Could you check a few things on this model? Use its own coordinates, in mm. Coordinates: 2 decimals unless noted, no trailing zeros. Order: outer loops, then holes, each group sorted by start corner. A loop starts at its lowest first (then second) coordinate and runs counter-clockwise, first axis right, second up. Notation, with made-up numbers: (39, 68) - (83, 68) arc R24 ccw to (83, 88) - close; hole circle Ø4 at (17.5, 39.25). An arc over 180 degrees is marked (long way). One line per item, written item: value. Start each with the question number.
from build123d import *

# Parameters (mm, degrees)
F0_R     = 13.75
F0_R_2   = 11.25
F1_DEPTH = 110
F4_R     = 5
F5_DEPTH = 33.751
F6_DEPTH = 33.751


with BuildPart() as f1:
    # F0 (on Front) → F1 (new body)
    with BuildSketch(Plane.XZ):
        Circle(F0_R)
        Circle(F0_R_2, mode=Mode.SUBTRACT)
    extrude(amount=F1_DEPTH)

    # F4 (on offset) → F5 (cut, through all)
    with BuildSketch(Plane.XY.offset(-20)):
        with Locations((0, -30)):
            Circle(F4_R)
    extrude(amount=F5_DEPTH, mode=Mode.SUBTRACT)

    # F4 (on offset) → F6 (cut, through all)
    with BuildSketch(Plane.XY.offset(-20)):
        with BuildLine():
            Line((-21.2415, 7.674746), (-21.2415, -2.517288))
            Line((-21.2415, -2.517288), (-21.2415, -5.328869))
            ThreePointArc((-21.2415, -5.328869), (0.089579, -8.9e-05), (21.399274, -5.413752))
            Line((21.399274, -5.413752), (21.399274, -2.555365))
            Line((21.399274, -2.555365), (21.399274, 6.795851))
            Line((21.399274, 6.795851), (-21.2415, 7.674746))
        make_face()
    extrude(amount=F6_DEPTH, mode=Mode.SUBTRACT)


solid = f1.part
Q1. I'm going to push flat-ended pins straight in: pin 1 (2 mm diameter, centred on x = -9, y = -68.5, fed in from +Z); pin 2 (12 mm diameter, centred on x = 9.5, y = -94, fed in from +Z); pin 3 (8 mm diameter, centred on x = 7.5, z = -5.5, fed in from +Y); pin 4 (8 mm diameter, centred on x = 0, y = -30, fed in from +Z). Where does each tip first touch, or does it pass through?
Q2. I want a section at D-D on y = -10. Please give me the cut outline in (x, z).
Q3. We'd pull the mould along Y, two halves only. Please class faces 1 (the cylindrical face through (5.1, -0.29, -10.25)), 2 (the cylindrical face through (3, -26, -12)), 3 (the cylindrical face through (10.39, -54.23, -4.31)): +Y half, -Y half, draft (parallel to the pull), parting line (faces both ways), or undercut.
Q4. If I drill on L1, parallel to Y at x = 0, z = -12.4; L2, parallel to Z at x = 0, y = -51, over which ranges is the centre line in solid material (lowest first)?
Q5. I want a section at A-A on x = 0. Please give me the cut outline in (y, z), then the cut area to 3 significant figures.
Q6. I want a section at B-B on z = 6.25. Please give me the cut outline in (x, y).
Q7. I want a section at C-C on x = -9. Please give me the cut outline in (y, z), then the cut area to 3 significant figures.
Values follow:
1. pin 1: stops at z = 11.18
1. pin 2: stops at z = 13.3
1. pin 3: stops at y = -0.44
1. pin 4: passes through
2. outline: circle Ø27.5 at (0, 0); hole circle Ø22.5 at (0, 0)
3. face 1: +Y half
3. face 2: undercut
3. face 3: draft
4. L1: y = -110 to -35, -25 to 0
4. L2: z = -13.75 to -11.25, 11.25 to 13.75
5. outline: (-110, -13.75) - (-35, -13.75) - (-35, -11.25) - (-110, -11.25) - close; (-110, 11.25) - (-35, 11.25) - (-35, 13.75) - (-110, 13.75) - close; (-25, -13.75) - (0, -13.75) - (0, -11.25) - (-25, -11.25) - close; (-25, 11.25) - (0, 11.25) - (0, 13.75) - (-25, 13.75) - close
5. area: 500 mm^2
6. outline: (-12.25, -110) - (-9.35, -110) - (-9.35, -0.98) arc R45 ccw to (-12.25, -1.7) - close; (9.35, -110) - (12.25, -110) - (12.25, -1.7) arc R45 ccw to (9.35, -0.98) - close
7. outline: (-110, -10.4) - (-0.91, -10.4) - (-0.91, -6.75) - (-110, -6.75) - close; (-110, 6.75) - (-0.91, 6.75) - (-0.91, 10.4) - (-110, 10.4) - close
7. area: 795 mm^2
